Work out the finished part from the listing and answer in its coordinate system (mm). Face numbers are marked on the shaded views. A direction names the side the tool comes from. Round coordinates to 2 decimals unless told otherwise and drop trailing zeros. Write each loop counter-clockwise with the first axis right and the second up, starting at its lowest first coordinate (ties: lowest second). Pieces come first, ordered by that corner, then holes. Notation, with made-up numbers: (-24, 56) -> (27, 56) arc R18 ccw to (27, 85) -> close; hole circle Ø6 at (-39.5, -20.5). An arc over 180 degrees is marked (long way). Answer as a JSON object with one key per item and string values. Group by question number.
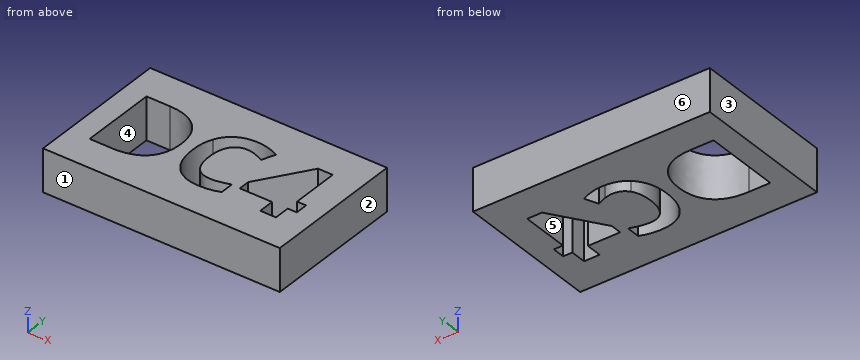
from build123d import *

# Parameters (mm, degrees)
F0_W     = 139.312
F0_H     = 84.13
F1_DEPTH = 25


with BuildPart() as f1:
    # F0 (on Top) → F1 (new body)
    with BuildSketch(Plane.XY):
        Rectangle(F0_W, F0_H)
        with BuildLine():
            add(Edge.make_bspline(
                [(-25.8895429555, 16.2212613242), (-19.8561711311, 10.4656780249), (-19.8561711311, 0.1338942869)],
                knots=[0, 0, 0, 1, 1, 1], degree=2))
            add(Edge.make_bspline(
                [(-19.8561711311, 0.1338942869), (-19.8561711311, -10.8606831248), (-26.1185966515, -16.7088625991)],
                knots=[0, 0, 0, 1, 1, 1], degree=2))
            add(Edge.make_bspline(
                [(-26.1185966515, -16.7088625991), (-32.381022172, -22.5570420735), (-44.1943447101, -22.5570420735)],
                knots=[0, 0, 0, 1, 1, 1], degree=2))
            Line((-44.1943447101, -22.5570420735), (-56.806918443, -22.5570420735))
            Line((-56.806918443, -22.5570420735), (-56.806918443, 21.9768446235))
            Line((-56.806918443, 21.9768446235), (-42.8297694994, 21.9768446235))
            add(Edge.make_bspline(
                [(-42.8297694994, 21.9768446235), (-31.9229147798, 21.9768446235), (-25.8895429555, 16.2212613242)],
                knots=[0, 0, 0, 1, 1, 1], degree=2))
        make_face(mode=Mode.SUBTRACT)
        with BuildLine():
            add(Edge.make_bspline(
                [(13.2542716593, 13.8722425686), (10.7298075196, 14.7543429727), (8.2930660719, 14.7543429727)],
                knots=[0, 0, 0, 1, 1, 1], degree=2))
            add(Edge.make_bspline(
                [(8.2930660719, 14.7543429727), (2.9614757845, 14.7543429727), (0.0373860474, 10.7483400328)],
                knots=[0, 0, 0, 1, 1, 1], degree=2))
            add(Edge.make_bspline(
                [(0.0373860474, 10.7483400328), (-2.8867036898, 6.7423370929), (-2.8867036898, -0.4119357974)],
                knots=[0, 0, 0, 1, 1, 1], degree=2))
            add(Edge.make_bspline(
                [(-2.8867036898, -0.4119357974), (-2.8867036898, -15.3052995253), (8.2930660719, -15.3052995253)],
                knots=[0, 0, 0, 1, 1, 1], degree=2))
            add(Edge.make_bspline(
                [(8.2930660719, -15.3052995253), (12.9813566172, -15.3052995253), (19.6482812179, -12.9660277356)],
                knots=[0, 0, 0, 1, 1, 1], degree=2))
            Line((19.6482812179, -12.9660277356), (19.6482812179, -20.8805639575))
            add(Edge.make_bspline(
                [(19.6482812179, -20.8805639575), (14.1704864436, -23.1711009183), (7.406092185, -23.1711009183)],
                knots=[0, 0, 0, 1, 1, 1], degree=2))
            add(Edge.make_bspline(
                [(7.406092185, -23.1711009183), (-2.3116327082, -23.1711009183), (-7.4580306456, -17.274186615)],
                knots=[0, 0, 0, 1, 1, 1], degree=2))
            add(Edge.make_bspline(
                [(-7.4580306456, -17.274186615), (-12.604428583, -11.3772723117), (-12.604428583, -0.3534540026)],
                knots=[0, 0, 0, 1, 1, 1], degree=2))
            add(Edge.make_bspline(
                [(-12.604428583, -0.3534540026), (-12.604428583, 6.596132606), (-10.0750909603, 11.8205062697)],
                knots=[0, 0, 0, 1, 1, 1], degree=2))
            add(Edge.make_bspline(
                [(-10.0750909603, 11.8205062697), (-7.5457533377, 17.0448799335), (-2.8087279635, 19.8276386667)],
                knots=[0, 0, 0, 1, 1, 1], degree=2))
            add(Edge.make_bspline(
                [(-2.8087279635, 19.8276386667), (1.9282974107, 22.6103973999), (8.2930660719, 22.6103973999)],
                knots=[0, 0, 0, 1, 1, 1], degree=2))
            add(Edge.make_bspline(
                [(8.2930660719, 22.6103973999), (14.7747983226, 22.6103973999), (21.3247593339, 19.4816213811)],
                knots=[0, 0, 0, 1, 1, 1], degree=2))
            Line((21.3247593339, 19.4816213811), (18.2837060072, 11.8010123382))
            add(Edge.make_bspline(
                [(18.2837060072, 11.8010123382), (15.7787357991, 12.9901421646), (13.2542716593, 13.8722425686)],
                knots=[0, 0, 0, 1, 1, 1], degree=2))
        make_face(mode=Mode.SUBTRACT)
        Polygon((58.1487960905, -6.0164411269), (58.1487960905, -13.3266654698), (52.7879649057, -13.3266654698), (52.7879649057, -22.5570420735), (43.5868291994, -22.5570420735), (43.5868291994, -13.3266654698), (24.5802459079, -13.3266654698), (24.5802459079, -6.7767044586), (44.1131653521, 21.9768446235), (52.7879649057, 21.9768446235), (52.7879649057, -6.0164411269), align=None, mode=Mode.SUBTRACT)
    extrude(amount=F1_DEPTH)


solid = f1.part
1) A cutting plane is placed at B-B on y = -18.5. State how many separate pieces and enclosed holes the cut face has, plus the area to 3 significant figures.
2) A cutting plane is placed at A-A on x = 40.5. Determine the outline of the cut face in (y, z) (3 decimals), plus the area to 3 significant figures.
3) Straight lines are drawn through the part: L1, parallel to X at y = -16, z = 13.5; L2, parallel to Y at x = 7, z = 3 (1 decimal); L3, parallel to Y at x = 56.5, z = 12.75 (3 decimals). For each, find the intervals that lie inside material, in ascending order.
4) A tool of negligible diameter and unlimited length cuts with its end or side. For the marked faces 5 and 6, from which of +Z, -Z, +X, -X, +Y, -Y can it reach the whole face along a straight path? Write none if from no direction.
5) For a pull along X with two mould halves and no side action, classify the marked faces 1, 2, 3 and 4 as released by +X, released by -X, zero draft, split by the parting line, or undercut.
6) This flat-tipped pin is pushed along its axis until it touches: P1, Ø8, axis at x = -7, y = 33.5, coming from the -Z side. Where does it stop, or does it pass through?
Established:
{
 "1": {"separate pieces": "4", "enclosed holes": "0", "area": "1,890 mm²"},
 "2": {"outline": "(-42.065, 0) -> (-13.327, 0) -> (-13.327, 25) -> (-42.065, 25) -> close; (16.658, 0) -> (42.065, 0) -> (42.065, 25) -> (16.658, 25) -> close", "area": "1,350 mm²"},
 "3": {"L1": "x = -69.66 to -56.81, -25.4 to -8.47, 19.65 to 43.59, 52.79 to 69.66", "L2": "y = -42.1 to -23.2, -15.3 to 14.7, 22.6 to 42.1", "L3": "y = -42.065 to -13.327, -6.016 to 42.065"},
 "4": {"face 5": "+Z, -Z", "face 6": "+Z, -Z, +X, -X, +Y"},
 "5": {"face 1": "zero draft", "face 2": "released by +X", "face 3": "released by -X", "face 4": "undercut"},
 "6": {"P1": "stops at z = 0"}
}
